Work out the finished part from the listing and answer in its coordinate system (mm). Give positions to 0.01 mm unless a question says otherwise; leave off trailing zeros. Order: outer loops, then holes, each group sorted by start corner. A loop starts at its lowest first (then second) coordinate and runs counter-clockwise, first axis right, second up.
```python
from build123d import *

# Parameters (mm, degrees)
SKETCH_1_W          = 450
SKETCH_1_H          = 20
EXTRUDE_1_DEPTH     = 30
SKETCH_2_R          = 7.5
CUT_EXTRUDE_1_DEPTH = 30
SKETCH_3_R          = 5
CUT_EXTRUDE_2_DEPTH = 228.870577302


with BuildPart() as part:
    # 草图1 → 凸台-拉伸1 (new body)
    with BuildSketch(Plane.XY):
        Rectangle(SKETCH_1_W, SKETCH_1_H)
    extrude(amount=EXTRUDE_1_DEPTH)

    # 草图2 → 切除-拉伸1 (cut)
    with BuildSketch(Plane(origin=(0, 10, 0), x_dir=(1, 0, 0), z_dir=(0, 1, 0))):
        with Locations(Location((-205, -15, 0), (0, 0, 270))):
            Circle(SKETCH_2_R)
    extrude(amount=-CUT_EXTRUDE_1_DEPTH, mode=Mode.SUBTRACT)

    # 草图3 → 切除-拉伸2 (cut, through all)
    with BuildSketch(Plane(origin=(0, 10, 0), x_dir=(1, 0, 0), z_dir=(0, 1, 0))):
        with Locations(Location((200, -15, 0), (0, 0, 270))):
            Circle(SKETCH_3_R)
    extrude(amount=-CUT_EXTRUDE_2_DEPTH, mode=Mode.SUBTRACT)


solid = part.part
```
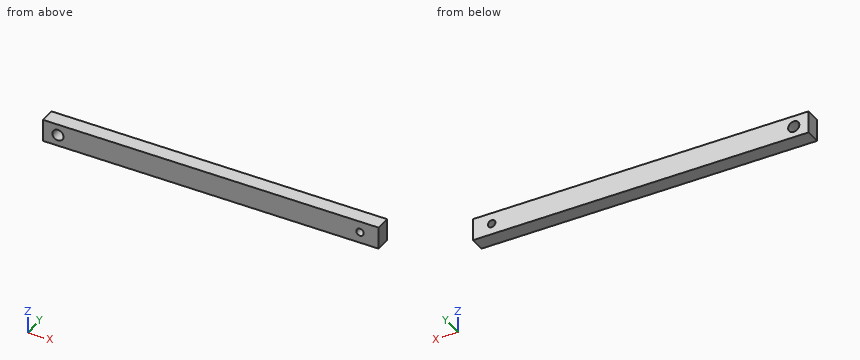
1. Given P1, Ø9, axis at x = -205, z = 15, coming from the +Y side, flat-ended and moving along its own axis, determine where the tip first touches the part or whether it passes through.
Findings below:
P1: passes through
2. The part is cut by section B-B (x = 200). Write down the section's boundary in (y, z).
Findings below:
outline: (-10, 0) - (10, 0) - (10, 10) - (-10, 10) - close; (-10, 20) - (10, 20) - (10, 30) - (-10, 30) - close
3. The part is cut by section C-C (x = -205). Write down the section's boundary in (y, z).
Findings below:
outline: (-10, 0) - (10, 0) - (10, 7.5) - (-10, 7.5) - close; (-10, 22.5) - (10, 22.5) - (10, 30) - (-10, 30) - close
4. The part is cut by section A-A (z = 15). Write down the section's boundary in (x, y), then the cut area to 3 significant figures.
Findings below:
outline: (-225, -10) - (-212.5, -10) - (-212.5, 10) - (-225, 10) - close; (-197.5, -10) - (195, -10) - (195, 10) - (-197.5, 10) - close; (205, -10) - (225, -10) - (225, 10) - (205, 10) - close
area: 8,500 mm2
5. Straight lines are drawn through the part: probe 1 along X at (y, z) = (3.5, 15); probe 2 along Z at (x, y) = (-199.5, 4.5); probe 3 along X at (y, z) = (-3, 21). For each, find the intervals that lie inside material, in ascending order.
Findings below:
probe 1: x = -225 to -212.5, -197.5 to 195, 205 to 225
probe 2: z = 0 to 9.9, 20.1 to 30
probe 3: x = -225 to -209.5, -200.5 to 225
